Source: CAD feature listing. Evaluate the final solid. Frame: model axes, mm. A direction names the side the tool comes from. Give positions to 0.01 mm unless a question says otherwise; leave off trailing zeros. Write each loop counter-clockwise with the first axis right and the second up, starting at its lowest first coordinate (ties: lowest second). Pieces come first, ordered by that corner, then holes. Notation, with made-up numbers: (-17.5, 85) - (18.5, 85) arc R11 ccw to (18.5, 103) - close; hole circle Ø5 at (-15, 71). An arc over 180 degrees is marked (long way). One line per question, with ' | ' between items. Start each with the question number.
(1) Draft query along Z for faces 1 (the flat face through (49, 63.077, 0)), 2 (the cylindrical face through (48.57, 60.12, 0.94)), 3 (the flat face through (15, 76, 12.5)). Return one class per face: +Z half, -Z half, draft (parallel to the pull), parting line (faces both ways), or undercut.
(2) Section C-C, the plane z = 0. Return loops of the section in (x, y), plus the area to 3 significant figures.
(3) Pin query (flat end, axial travel): pin 1 (5 mm diameter, centred on y = 66, z = 0, fed in from +X); pin 2 (6 mm diameter, centred on y = 84, z = 3.5, fed in from -X); pin 3 (10 mm diameter, centred on y = 66, z = 2, fed in from +X); pin 4 (3 mm diameter, centred on x = 47.09, z = 0, fed in from -Y). Return the tip coordinate at first contact, or that it passes through.
(4) Access query for faces 4 (the flat face through (7.397, 66, 0)), 5 (the cylindrical face through (39.567, 57.678, 0.175)), 6 (the cylindrical face through (1.553, 60.119, 8.358)), 7 (the flat face through (44.997, 66, 0)). Directions: +Z, -Z, +X, -X, +Y, -Y. A direction counts if a zero-diameter tool reaches every point of the face in a straight line with its end or side. Return the directions, or none.
(5) Ray query, line 1 (X direction, y = 65, z = -5.25); line 2 (X direction, y = 62, z = 5.75); line 3 (X direction, y = 81, z = 10.75). Return the intervals inside material, ascending. Write a range as [from, to].
(6) Section A-A, the plane z = -6.25. Return loops of the section in (x, y), plus the area to 3 significant figures.
(7) Section B-B, the plane y = 71. Return loops of the section in (x, z), plus the area to 3 significant figures.
(8) Section D-D, the plane y = 75.5. Return loops of the section in (x, z), plus the area to 3 significant figures.
```python
from build123d import *

# Parameters (mm, degrees)
BOSS_EXTRU_1_DEPTH      = 12.5
ESQUISSE2_R             = 2.5
ESQUISSE2_R_2           = 1.75
ENL_V_MAT_EXTRU_1_DEPTH = 10
CONG_4_R                = 3
CONG_5_R                = 1.5


with BuildPart() as part:
    # Esquisse1 → Boss.-Extru.1 (new, symmetric)
    with BuildSketch(Plane.XY):
        with BuildLine():
            Line((0.397051683, 57.076719782), (10.397051683, 57.076719782))
            ThreePointArc((10.397051683, 57.076719782), (12.518372027, 57.955399438), (13.397051683, 60.076719782))
            Line((13.397051683, 60.076719782), (13.397051683, 69.276719782))
            ThreePointArc((13.397051683, 69.276719782), (26.197051683, 82.076719782), (38.997051683, 69.276719782))
            Line((38.997051683, 69.276719782), (38.997051683, 59.076719782))
            ThreePointArc((38.997051683, 59.076719782), (39.582838121, 57.662506219), (40.997051683, 57.076719782))
            Line((40.997051683, 57.076719782), (49.420552909, 57.076719782))
            Line((49.420552909, 57.076719782), (52.447260314, 57.076719782))
            Line((52.447260314, 57.076719782), (52.447260314, 63.076719782))
            Line((52.447260314, 63.076719782), (49.420552909, 63.076719782))
            Line((49.420552909, 63.076719782), (44.997051683, 63.076719782))
            Line((44.997051683, 63.076719782), (44.997051683, 69.276719782))
            ThreePointArc((44.997051683, 69.276719782), (26.197051683, 88.076719782), (7.397051683, 69.276719782))
            Line((7.397051683, 69.276719782), (7.397051683, 63.076719782))
            Line((7.397051683, 63.076719782), (0.397051683, 63.076719782))
            Line((0.397051683, 63.076719782), (-1.602948317, 63.076719782))
            Line((-1.602948317, 63.076719782), (-1.602948317, 57.076719782))
            Line((-1.602948317, 57.076719782), (0.397051683, 57.076719782))
        make_face()
    extrude(amount=BOSS_EXTRU_1_DEPTH, both=True)

    # Esquisse2 → Enlèv. mat.-Extru.1 (cut)
    with BuildSketch(Plane(origin=(0, 63.076719782, 0), x_dir=(1, 0, 0), z_dir=(0, 1, 0))):
        with Locations(Location((2.897051683, 6.25, 0), (0, 0, 270))):
            Circle(ESQUISSE2_R)
        with Locations(Location((2.897051683, -6.25, 0), (0, 0, 180))):
            Circle(ESQUISSE2_R)
        with Locations(Location((47.0933932, 0, 0), (0, 0, 270))):
            Circle(ESQUISSE2_R_2)
    extrude(amount=-ENL_V_MAT_EXTRU_1_DEPTH, mode=Mode.SUBTRACT)

    # Congé4
    cong_4_edges = [part.edges().sort_by_distance(p)[0] for p in [
        (52.447260314, 63.076719782, 0),
    ]]
    fillet(cong_4_edges, radius=CONG_4_R)

    # Congé5
    cong_5_edges = [part.edges().sort_by_distance(p)[0] for p in [
        (-1.602948317, 63.076719782, 0),
    ]]
    fillet(cong_5_edges, radius=CONG_5_R)


solid = part.part
```
Check sheet entries:
1) face 1: draft | face 2: undercut | face 3: +Z half
2) outline: (-1.6, 57.08) - (10.4, 57.08) arc R3 ccw to (13.4, 60.08) - (13.4, 69.28) arc R12.8 cw to (39, 69.28) - (39, 59.08) arc R2 ccw to (41, 57.08) - (45.34, 57.08) - (45.34, 63.08) - (45, 63.08) - (45, 69.28) arc R18.8 ccw to (7.4, 69.28) - (7.4, 63.08) - (-0.1, 63.08) arc R1.5 ccw to (-1.6, 61.58) - close; (48.84, 57.08) - (52.45, 57.08) - (52.45, 60.08) arc R3 ccw to (49.45, 63.08) - (48.84, 63.08) - close | area: 517 mm²
3) pin 1: x = 45 | pin 2: x = 11.5 | pin 3: x = 52.3 | pin 4: through
4) face 4: +Z, -Z, -X, +Y | face 5: +Z, -Z, -Y | face 6: +Y, -Y | face 7: +Z, -Z, +X, +Y
5) line 1: [7.4, 13.4], [39, 45] | line 2: [-1.54, 0.45], [5.35, 13.4], [39, 51.75] | line 3: [11.5, 21.06], [31.34, 40.89]
6) outline: (-1.6, 57.08) - (0.4, 57.08) - (0.4, 63.08) - (-0.1, 63.08) arc R1.5 ccw to (-1.6, 61.58) - close; (5.4, 57.08) - (10.4, 57.08) arc R3 ccw to (13.4, 60.08) - (13.4, 69.28) arc R12.8 cw to (39, 69.28) - (39, 59.08) arc R2 ccw to (41, 57.08) - (52.45, 57.08) - (52.45, 60.08) arc R3 ccw to (49.45, 63.08) - (45, 63.08) - (45, 69.28) arc R18.8 ccw to (7.4, 69.28) - (7.4, 63.08) - (5.4, 63.08) - close | area: 508 mm²
7) outline: (7.48, -12.5) - (13.51, -12.5) - (13.51, 12.5) - (7.48, 12.5) - close; (38.88, -12.5) - (44.92, -12.5) - (44.92, 12.5) - (38.88, 12.5) - close | area: 302 mm²
8) outline: (8.46, -12.5) - (15.01, -12.5) - (15.01, 12.5) - (8.46, 12.5) - close; (37.38, -12.5) - (43.94, -12.5) - (43.94, 12.5) - (37.38, 12.5) - close | area: 328 mm²
